Verification items for the finished model (mm, model axes). A direction names the side the tool comes from. Give positions to 0.01 mm unless a question says otherwise; leave off trailing zeros. Answer as a JSON object with one key per item and string values.
```python
from build123d import *

# Parameters (mm, degrees)
SZKIC1_W                                            = 220
SZKIC1_H                                            = 237
DODANIE_WYCI_GNI_CIE1_DEPTH                         = 5
POG_BIENIE_WALCOWE_POD_M3_WKR_T_Z_BEM_W_D           = 3.6
POG_BIENIE_WALCOWE_POD_M3_WKR_T_Z_BEM_W_DEPTH       = 6.7
POG_BIENIE_WALCOWE_POD_M3_WKR_T_Z_BEM_W_CBORE_D     = 6.5
POG_BIENIE_WALCOWE_POD_M3_WKR_T_Z_BEM_W_CBORE_DEPTH = 3.4
POG_BIENIE_WALCOWE_POD_M3_WKR_T_Z_BEM_W_TIP         = 1.081549114


with BuildPart() as part:
    # Szkic1 → Dodanie-wyciągnięcie1 (new body)
    with BuildSketch(Plane.XY):
        Rectangle(SZKIC1_W, SZKIC1_H)
    extrude(amount=DODANIE_WYCI_GNI_CIE1_DEPTH)

    # Pogłębienie walcowe pod M3 Wkręt z łbem walcowym z gniazdem1
    with Locations(Plane.XY.offset(5)):
        with Locations((105, -115), (105, 115), (-105, 115), (-105, -115)):
            CounterBoreHole(POG_BIENIE_WALCOWE_POD_M3_WKR_T_Z_BEM_W_D / 2, POG_BIENIE_WALCOWE_POD_M3_WKR_T_Z_BEM_W_CBORE_D / 2, POG_BIENIE_WALCOWE_POD_M3_WKR_T_Z_BEM_W_CBORE_DEPTH, depth=POG_BIENIE_WALCOWE_POD_M3_WKR_T_Z_BEM_W_DEPTH)
            with Locations((0, 0, -(POG_BIENIE_WALCOWE_POD_M3_WKR_T_Z_BEM_W_DEPTH + POG_BIENIE_WALCOWE_POD_M3_WKR_T_Z_BEM_W_TIP / 2))):  # 118° drill point
                Cone(0, POG_BIENIE_WALCOWE_POD_M3_WKR_T_Z_BEM_W_D / 2, POG_BIENIE_WALCOWE_POD_M3_WKR_T_Z_BEM_W_TIP, mode=Mode.SUBTRACT)


solid = part.part
```
1) Access from +Z, -Z, +X, -X, +Y, -Y to the whole of each face (thin tool, end or side, straight path). Record for faces 4 (the face through (-2, -118.5, 2)), 5 (the face through (-105.705, -118.173, 3.324)).
Completed:
{"face 4": "+Z, -Z, +X, -X, -Y", "face 5": "+Z"}
2) Release check for a two-part mould opening along Y. For faces 1 (the face through (104.295, 111.827, 3.324)), 2 (the face through (-110, -2, 2)), 3 (the face through (-2, 118.5, 2)) record: pulls with the +Y half, pulls with the -Y half, needs draft (parallel to the pull), parting line crosses it, or undercut.
Completed:
{"face 1": "undercut", "face 2": "needs draft", "face 3": "pulls with the +Y half"}
3) Go/stop test with flat-tipped pins: pin 1 (3 mm diameter, centred on x = -105, y = 115, fed in from +Z); pin 2 (3 mm diameter, centred on x = 105, y = 116, fed in from +Z). Record where each tip stops, or that it passes through.
Completed:
{"pin 1": "passes through", "pin 2": "stops at z = 1.6"}
4) Thickness scan on L1, parallel to X at y = -115, z = 1.2; L2, parallel to Y at x = 105, z = 0.95; L3, parallel to Y at x = -105, z = 3. Record the ranges inside material, lowest first.
Completed:
{"L1": "x = -110 to -106.8, -103.2 to 103.2, 106.8 to 110", "L2": "y = -118.5 to -116.8, -113.2 to 113.2, 116.8 to 118.5", "L3": "y = -118.5 to -118.25, -111.75 to 111.75, 118.25 to 118.5"}
